Verification items for the finished model (mm, model axes). A direction names the side the tool comes from. Give positions to 0.01 mm unless a question says otherwise; leave off trailing zeros. Loops run counter-clockwise (first coordinate to the right, second up) from the corner with the lowest first, then second, coordinate; pieces in that order, holes last. Notation, with made-up numbers: (-22, -1) - (30, -1) arc R26 ccw to (30, 21) - close; hole circle Ø1 at (-9.75, -32). An arc over 180 degrees is marked (long way). Answer in a Markdown table with one row per item.
```python
from build123d import *

# Parameters (mm, degrees)
SKETCH_W        = 1600
SKETCH_H        = 800
PAD_DEPTH       = 900
SKETCH001_W     = 1399.489502
SKETCH001_H     = 357.799927
SKETCH001_W_2   = 1411.382736
SKETCH001_H_2   = 386.889557
POCKET_DEPTH    = 800
SKETCH002_W     = 648.389411
SKETCH002_H     = 831.100419
POCKET001_DEPTH = 5
SKETCH003_W     = 623.226656
SKETCH003_H     = 886.54245
POCKET002_DEPTH = 5
SKETCH004_W     = 249.06694
SKETCH004_H     = 318.805694
SKETCH004_W_2   = 215.858154
SKETCH004_H_2   = 313.345032
SKETCH004_W_3   = 252.387802
SKETCH004_H_3   = 262.350571
SKETCH004_W_4   = 209.216248
SKETCH004_H_4   = 262.099701
POCKET003_DEPTH = 5
SKETCH005_W     = 263.345154
SKETCH005_H     = 305.770508
SKETCH005_W_2   = 235.499115
SKETCH005_H_2   = 306.489624
SKETCH005_W_3   = 259.166199
SKETCH005_H_3   = 340.773849
SKETCH005_W_4   = 237.131774
SKETCH005_H_4   = 326.798797
POCKET004_DEPTH = 5


with BuildPart() as part:
    # Sketch → Pad (new body)
    with BuildSketch(Plane.XZ):
        with Locations((800, 400)):
            Rectangle(SKETCH_W, SKETCH_H)
    extrude(amount=PAD_DEPTH)

    # Sketch001 (on Face6 of Pad) → Pocket (cut)
    with BuildSketch(Plane.XZ.offset(900)):
        with Locations((799.744751, 671.889404)):
            Rectangle(SKETCH001_W, SKETCH001_H)
        with Locations((798.594947, 93.649276)):
            Rectangle(SKETCH001_W_2, SKETCH001_H_2)
    extrude(amount=-POCKET_DEPTH, mode=Mode.SUBTRACT)

    # Sketch002 (on Face8 of Pocket) → Pocket001 (cut)
    with BuildSketch(Plane(origin=(0, 0, 0), x_dir=(0, 0, -1), z_dir=(-1, 0, 0))):
        with Locations((-404.729881, 532.556495)):
            Rectangle(SKETCH002_W, SKETCH002_H)
    extrude(amount=-POCKET001_DEPTH, mode=Mode.SUBTRACT)

    # Sketch003 (on Face3 of Pocket001) → Pocket002 (cut)
    with BuildSketch(Plane(origin=(1600, 0, 0), x_dir=(0, 0, 1), z_dir=(1, 0, 0))):
        with Locations((401.204392, 568.800241)):
            Rectangle(SKETCH003_W, SKETCH003_H)
    extrude(amount=-POCKET002_DEPTH, mode=Mode.SUBTRACT)

    # Sketch004 (on Face14 of Pocket002) → Pocket003 (cut)
    with BuildSketch(Plane(origin=(1595, 0, 0), x_dir=(0, 0, 1), z_dir=(1, 0, 0))):
        with Locations((263.843483, 640.951462)):
            Rectangle(SKETCH004_W, SKETCH004_H)
        with Locations((552.92334, 641.542023)):
            Rectangle(SKETCH004_W_2, SKETCH004_H_2)
        with Locations((265.503914, 297.23899)):
            Rectangle(SKETCH004_W_3, SKETCH004_H_3)
        with Locations((550.027313, 297.826859)):
            Rectangle(SKETCH004_W_4, SKETCH004_H_4)
    extrude(amount=-POCKET003_DEPTH, mode=Mode.SUBTRACT)

    # Sketch005 (on Face19 of Pocket003) → Pocket004 (cut)
    with BuildSketch(Plane(origin=(5, 0, 0), x_dir=(0, 0, -1), z_dir=(-1, 0, 0))):
        with Locations((-563.361725, 704.925354)):
            Rectangle(SKETCH005_W, SKETCH005_H)
        with Locations((-248.631547, 700.386841)):
            Rectangle(SKETCH005_W_2, SKETCH005_H_2)
        with Locations((-561.272247, 326.141334)):
            Rectangle(SKETCH005_W_3, SKETCH005_H_3)
        with Locations((-249.447876, 323.332688)):
            Rectangle(SKETCH005_W_4, SKETCH005_H_4)
    extrude(amount=-POCKET004_DEPTH, mode=Mode.SUBTRACT)


solid = part.part
```
Q1. Sectioned sample at B-B (y = -819.5). Record the cut outline in (x, z).
Completed:
| item | result |
|---|---|
| outline | (0, 0) - (92.9, 0) - (92.9, 287.09) - (1504.29, 287.09) - (1504.29, 0) - (1600, 0) - (1600, 89.59) - (1595, 89.59) - (1595, 712.82) - (1600, 712.82) - (1600, 800) - (1499.49, 800) - (1499.49, 492.99) - (100, 492.99) - (100, 800) - (0, 800) - (0, 728.92) - (5, 728.92) - (5, 695.03) - (10, 695.03) - (10, 431.69) - (5, 431.69) - (5, 366.38) - (10, 366.38) - (10, 130.88) - (5, 130.88) - (5, 80.54) - (0, 80.54) - close |
Q2. Go/stop test with flat-tipped pins: P1, Ø1, axis at x = 397, z = 148.5, coming from the -Y side; P2, Ø12, axis at x = 1369.5, y = -649.5, coming from the -Z side; P3, Ø1, axis at y = -602, z = 304, coming from the +X side. Record where each tip stops, or that it passes through.
Completed:
| item | result |
|---|---|
| P1 | y = -100 |
| P2 | z = 287.09 |
| P3 | x = 1590 |
Q3. Sectioned sample at A-A (z = 242). Record the cut outline in (x, y), and give its area (3 significant figures).
Completed:
| item | result |
|---|---|
| outline | (0, -117.01) - (5, -117.01) - (5, -159.93) - (10, -159.93) - (10, -486.73) - (5, -486.73) - (5, -547.14) - (10, -547.14) - (10, -853.63) - (5, -853.63) - (5, -900) - (92.9, -900) - (92.9, -100) - (1504.29, -100) - (1504.29, -900) - (1595, -900) - (1595, -800.35) - (1590, -800.35) - (1590, -481.55) - (1595, -481.55) - (1595, -428.41) - (1590, -428.41) - (1590, -166.06) - (1595, -166.06) - (1595, -125.53) - (1600, -125.53) - (1600, 0) - (0, 0) - close |
| area | 297,000 mm^2 |
Q4. Draft check along Y on faces 1 (the face through (10, -329, 563)), 2 (the face through (1504.286, -506, 142)), 3 (the face through (789, 0, 406)). Enter one of: +Y half, -Y half, draft (parallel to the pull), parting line (faces both ways), or undercut.
Completed:
| item | result |
|---|---|
| face 1 | undercut |
| face 2 | draft |
| face 3 | +Y half |
Q5. Thickness scan on line 1 (X direction, y = -388, z = 85.5); line 2 (X direction, y = -659.5, z = 632); line 3 (Z direction, x = 884, y = -208). Record the ranges inside material, lowest first.
Completed:
| item | result |
|---|---|
| line 1 | 5 to 92.9, 1504.29 to 1600 |
| line 2 | 10 to 100, 1499.49 to 1590 |
| line 3 | 287.09 to 492.99 |
Q6. Tool access check on faces 4 (the face through (790, -506, 492.989)), 5 (the face through (789, -100, 146)), 6 (the face through (10, -326, 251)). Record the directions out of +Z, -Z, +X, -X, +Y, -Y that give a thin tool (end or side, any length) a straight path to the whole face; none if there is none.
Completed:
| item | result |
|---|---|
| face 4 | +Z, -Y |
| face 5 | -Z, -Y |
| face 6 | -X |
Q7. Sectioned sample at C-C (x = 731). Record the cut outline in (y, z), and give its area (3 significant figures).
Completed:
| item | result |
|---|---|
| outline | (-900, 287.09) - (-100, 287.09) - (-100, 0) - (0, 0) - (0, 800) - (-100, 800) - (-100, 492.99) - (-900, 492.99) - close |
| area | 245,000 mm^2 |
